Autodesk Inventor part; units mm, degrees
ref_plane "XZ Plane" through (0, 0, 0) normal (0, 1, 0) x (-1, 0, 0)
sketch "Sketch1" plane through (0, 0, 0) normal (0, 0, 1) x (1, 0, 0)
  line L0 (-18, 0) -> (-18, 10)
  line L1 (-18, 10) -> (-20, 10)
  line L2 (-20, 10) -> (-20, 12.5)
  line L3 (-20, 12.5) -> (-15, 12.5)
  line L4 (-15, 12.5) -> (-15, 15)
  line L5 (-15, 15) -> (-20, 15)
  line L6 (-20, 15) -> (-20, 17.5)
  line L7 (-20, 17.5) -> (-15, 17.5)
  line L8 (-15, 17.5) -> (-15, 20)
  line L9 (-15, 20) -> (-20, 20)
  line L10 (-20, 20) -> (-20, 30)
  line L11 (-20, 30) -> (0, 30)
  line L12 (0, 30) -> (0, 0)
  line L13 (-18, 0) -> (-12, 0)
  line L14 (-12, 5) -> (-2, 5)
  line L15 (-12, 0) -> (-18, 0)
  line L16 (-2, -25) -> (0, -25)
  line L17 (0, 0) -> (0, -25)
  line L18 (-2, 5) -> (-2, -25)
  line L19 (-12, 5) -> (-12, 0)
  dimension "d0" = 2.5
  dimension "d1" = 20
  dimension "d3" = 5
  dimension "d4" = 10
  dimension "d22" = 10
  dimension "d24" = 30
  dimension "d26" = 2
  dimension "d27" = 25
  dimension "d28" = 10
  dimension "d29" = 30
  dimension "d30" = 18
revolve "Revolution1" add sketch "Sketch1" angle 360 about axis through (0, 30, 0) along (0, -1, 0)
ref_plane "Work Plane4" through (-20, 16.25, 0) normal (1, 0, 0) x (0, 1, 0)
sketch "Sketch6" plane through (-20, 16.25, 0) normal (1, 0, 0) x (0, 1, 0)
  line L0 (4.3754, -2.422) -> (10.3754, -2.422)
  line L1 (10.3754, -2.422) -> (10.3754, -0.6353)
  line L2 (10.3754, -0.6353) -> (4.3754, -0.6353)
  line L3 (4.3754, -0.6353) -> (4.3754, -2.422)
  line L4 (0.3754, -0.6353) -> (-5.6246, -0.6353)
  line L5 (-5.6246, -0.6353) -> (-5.6246, -2.422)
  line L6 (-5.6246, -2.422) -> (0.3754, -2.422)
  line L7 (0.3754, -2.422) -> (0.3754, -0.6353)
  line L8 (-830.9186, 0) -> (19.0814, 0)
  point P0 (0, 0)
  dimension "d39" = 6
  dimension "d40" = 6
  dimension "d41" = 10
  dimension "d42" = 1.7867
  dimension "d43" = 1.7867
  dimension "d44" = 10.3753
  dimension "d45" = 0.6353
  dimension "d46" = 0.6353
  dimension "d47" = 8.706
extrude "Extrusion2" add sketch "Sketch6" along normal blind 21.1125 and the other way blind 20.081
ref_plane "Work Plane5" through (0, 25, -20) normal (0, 0, 1) x (1, 0, 0)
sketch "Sketch7" plane through (0, 25, -20) normal (0, 0, 1) x (1, 0, 0)
  circle A0 centre (0, -20) radius 2.5
  point P0 (0, -25)
  dimension "d48" = 5
  dimension "d49" = 5
extrude "Extrusion3" add sketch "Sketch7" along normal blind 36.4625 and the other way blind 3.944
properties part number "BallHolder"
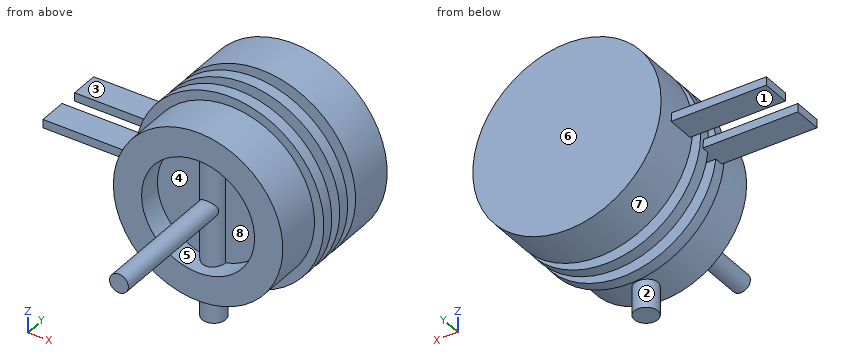
Input: part model. Units: mm. Frame: model coordinates. Face numbers are marked on the shaded views. A direction names the side the tool comes from. Coordinates: 2 decimals unless noted, no trailing zeros. Write each loop counter-clockwise with the first axis right and the second up, starting at its lowest first coordinate (ties: lowest second). Pieces come first, ordered by that corner, then holes.
1) Material intervals for line 1 along Z through (x, y) = (0, 2.25); line 2 along Y through (x, z) = (-12, 13.5), sorted ascending.
2) Section B-B on z = -13.5. Output: boundary loops of the cut face in (x, y).
3) Set-up query: the marked faces 1, 2, 3 and 4. Return all of +Z, -Z, +X, -X, +Y, -Y with unobstructed straight access to the full face (end or side cutting, diameter ignored); none if empty.
4) Pin query (flat end, axial travel): pin 1 Ø6.5 at (x, y) = (-33, 15) entering from -Z; pin 2 Ø2 at (x, z) = (-29.5, -1.5) entering from +Y; pin 3 Ø2 at (x, y) = (-17.5, 15) entering from +Z. Return the tip coordinate at first contact, or that it passes through.
5) Section C-C on x = 5. Output: boundary loops of the cut face in (y, z), and give its area (3 significant figures).
6) Mould query, pull axis X, two halves, no side actions, for the marked faces 5, 6, 7 and 8. Classes: pulls with the +X half, pulls with the -X half, needs draft (parallel to the pull), parting line crosses it, or undercut.
7) Section A-A on y = -7.5. Output: boundary loops of the cut face in (x, z).
Check result:
1. line 1: z = -18 to -12, -2 to 2, 12 to 18
1. line 2: y = 10 to 12.5, 15 to 17.5, 20 to 30
2. outline: (-14.76, 10) - (-11.91, 10) - (-11.91, 0) - (11.91, 0) - (11.91, 10) - (14.76, 10) - (14.76, 12.5) - (6.54, 12.5) - (6.54, 15) - (14.76, 15) - (14.76, 17.5) - (6.54, 17.5) - (6.54, 20) - (14.76, 20) - (14.76, 30) - (-14.76, 30) - (-14.76, 20) - (-6.54, 20) - (-6.54, 17.5) - (-14.76, 17.5) - (-14.76, 15) - (-6.54, 15) - (-6.54, 12.5) - (-14.76, 12.5) - close
3. face 1: -Z, -X, +Y, -Y
3. face 2: -Z
3. face 3: +Z, -X, +Y, -Y
3. face 4: -Y
4. pin 1: stops at z = -2.42
4. pin 2: stops at y = 26.63
4. pin 3: stops at z = 11.3
5. outline: (0, -17.29) - (10, -17.29) - (10, -19.36) - (12.5, -19.36) - (12.5, -14.14) - (15, -14.14) - (15, -19.36) - (17.5, -19.36) - (17.5, -14.14) - (20, -14.14) - (20, -19.36) - (30, -19.36) - (30, 19.36) - (20, 19.36) - (20, 14.14) - (17.5, 14.14) - (17.5, 19.36) - (15, 19.36) - (15, 14.14) - (12.5, 14.14) - (12.5, 19.36) - (10, 19.36) - (10, 17.29) - (0, 17.29) - (0, 10.91) - (5, 10.91) - (5, -10.91) - (0, -10.91) - close
5. area: 959 mm2
6. face 5: undercut
6. face 6: needs draft
6. face 7: parting line crosses it
6. face 8: undercut
7. outline: circle Ø4 at (0, 0)
